Geometry: final body of the model. Coordinates: model frame, mm. Face numbers are marked on the shaded views. A direction names the side the tool comes from. Give positions to 0.01 mm unless a question says otherwise; leave off trailing zeros. Write each loop counter-clockwise with the first axis right and the second up, starting at its lowest first coordinate (ties: lowest second). Pieces come first, ordered by that corner, then holes. Notation, with made-up numbers: M 61,-39.75 L 67,-39.75 A14 cw 67,-12.75 Z; hole C 86.25,89 d11. An arc over 180 degrees is marked long. Use a Markdown table: item, result. Add a question column.
1) Section C-C on x = -102.5. Return the cut outline in (y, z).
2) Line query: line 1 (Z direction, x = 0, y = 80); line 2 (Y direction, x = -79.5, z = -69.5); line 3 (X direction, y = 38.5, z = -42). Output: solid intervals per line, ascending.
3) Section A-A on z = -40.5. Return the cut outline in (x, y), then the cut area to 3 significant figures.
4) Section B-B on y = 17. Return the cut outline in (x, z), then the cut area to 3 significant figures.
5) Section D-D on z = -99.5. Return the cut outline in (x, y).
6) Pin query (flat end, axial travel): pin 1 (2 mm diameter, centred on y = 37.5, z = -42, fed in from -X); pin 2 (7.5 mm diameter, centred on x = -71.63, z = -2.45, fed in from -Y); pin 3 (12 mm diameter, centred on y = 24, z = -75.5, fed in from +X). Return the tip coordinate at first contact, or that it passes through.
7) Set-up query: the marked faces 1 and 2. Return all of +Z, -Z, +X, -X, +Y, -Y with unobstructed straight access to the full face (end or side cutting, diameter ignored); none if empty.
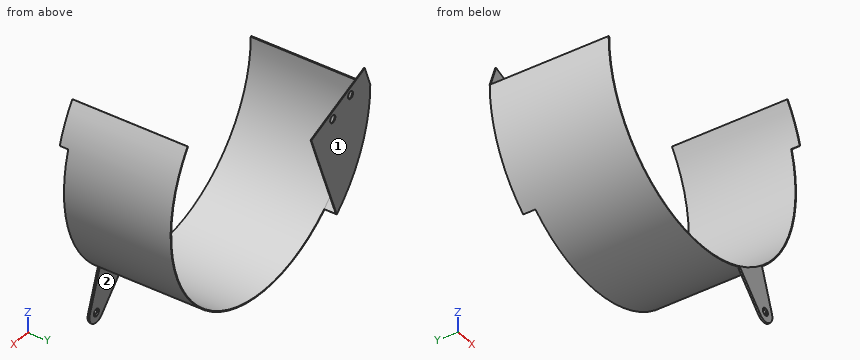
```python
from build123d import *
from build123d.topology import SkipClean

# Parameters (mm, degrees)
BASE_FLANGE1_DEPTH   = 102.87
CUT_EXTRUDE1_START   = -7.62
CUT_EXTRUDE1_DEPTH   = 7.62
BOSS_EXTRUDE5_START  = -95.25
BOSS_EXTRUDE5_DEPTH  = 95.25
BOSS_EXTRUDE6_DEPTH  = 10.16
BOSS_EXTRUDE7_DEPTH  = 0.762
SKETCH12_W           = 72.378245623
SKETCH12_H           = 0.762
BOSS_EXTRUDE8_DEPTH  = 20.33854962
SKETCH13_R           = 3.3
CUT_EXTRUDE2_DEPTH   = 204.597121983
SKETCH15_R           = 3.2639
BOSS_EXTRUDE10_DEPTH = 1.5875


# Read off the part's stored shape, not the designer's step: Cut-Extrude1
# Sheet-metal steps are written as plain solids
with BuildPart() as part:
    # Sketch2 → Base-Flange1 (new body)
    with BuildSketch(Plane(origin=(0, 0, 0), x_dir=(1, 0, 0), z_dir=(0, 1, 0))):
        with BuildLine():
            ThreePointArc((-119.38, 0), (35.898258345, 113.85472958), (97.790371047, -68.473554972))
            Line((97.790371047, -68.473554972), (97.186983651, -68.051058569))
            ThreePointArc((97.186983651, -68.051058569), (35.676758453, 113.152221674), (-118.6434, 0))
            Line((-118.6434, 0), (-119.38, 0))
        make_face()
    extrude(amount=BASE_FLANGE1_DEPTH)

    # Cut-Extrude1 outline → Cut-Extrude1 (cut)
    with BuildSketch(Plane.XZ.offset(CUT_EXTRUDE1_START)):
        with BuildLine():
            ThreePointArc((-119.38, 0), (18.160489843, -117.990597119), (113.85472958, 35.898258345))
            Line((113.85472958, 35.898258345), (113.152221674, 35.676758453))
            ThreePointArc((113.152221674, 35.676758453), (18.048435757, -117.262570031), (-118.6434, 0))
            Line((-118.6434, 0), (-119.38, 0))
        make_face()
    extrude(amount=CUT_EXTRUDE1_DEPTH, mode=Mode.SUBTRACT)

    # Sketch9 → Boss-Extrude5 (add)
    with BuildSketch(Plane(origin=(0, 102.87, 0), x_dir=(1, 0, 0), z_dir=(0, 1, 0)).offset(BOSS_EXTRUDE5_START)):
        with BuildLine():
            Line((-119.379693576, -0.270484204), (-118.6434, 0))
            Line((-118.6434, 0), (-119.38, 0))
            ThreePointArc((-119.38, 0), (-119.379923394, -0.135242189), (-119.379693576, -0.270484204))
        make_face()
    extrude(amount=BOSS_EXTRUDE5_DEPTH)

    # Sketch10 → Boss-Extrude6 (add)
    with SkipClean():  # the faces are left unmerged after this step: merging them gives an invalid solid
        with BuildSketch(Plane(origin=(0, 102.87, 0), x_dir=(1, 0, 0), z_dir=(0, 1, 0))):
            with BuildLine():
                Line((-119.379693576, -0.270484204), (-118.6434, 0))
                ThreePointArc((-118.6434, 0), (-107.527437301, 50.140867475), (-76.262507491, 90.886117283))
                Line((-76.262507491, 90.886117283), (-76.735984844, 91.45038562))
                ThreePointArc((-76.735984844, 91.45038562), (-108.252110006, 50.329564663), (-119.379693576, -0.270484204))
            make_face()
        extrude(amount=BOSS_EXTRUDE6_DEPTH)

    # Sketch11 → Boss-Extrude7 (add)
    with SkipClean():  # the faces are left unmerged after this step: merging them gives an invalid solid
        with BuildSketch(Plane(origin=(0, 113.03, 0), x_dir=(1, 0, 0), z_dir=(0, 1, 0))):
            with BuildLine():
                Line((-119.379693576, -0.270484204), (-51.440692331, 24.687531528))
                Line((-51.440692331, 24.687531528), (-76.735984844, 91.45038562))
                ThreePointArc((-76.735984844, 91.45038562), (-108.252110006, 50.329564663), (-119.379693576, -0.270484204))
            make_face()
        extrude(amount=BOSS_EXTRUDE7_DEPTH)

    # Sketch12 → Boss-Extrude8 (add)
    with SkipClean():  # the faces are left unmerged after this step: merging them gives an invalid solid
        with BuildSketch(Plane(origin=(-14.107419738, 0, -38.402251904), x_dir=(0.9386660406079884, 0, -0.3448275862069655), z_dir=(0.3448275862069655, 0, 0.9386660406079884))):
            with Locations((-75.961811901, 113.411)):
                Rectangle(SKETCH12_W, SKETCH12_H)
        extrude(amount=BOSS_EXTRUDE8_DEPTH)

    # Sketch13 → Cut-Extrude2 (cut, through all)
    with SkipClean():  # the faces are left unmerged after this step: merging them gives an invalid solid
        with BuildSketch(Plane(origin=(0, 113.792, 0), x_dir=(1, 0, 0), z_dir=(0, 1, 0))):
            with Locations(Location((-94.258662261, -5.860928581, 0), (0, 0, 270))):
                Circle(SKETCH13_R)
            with Locations(Location((-71.633967235, 2.450493285, 0), (0, 0, 270))):
                Circle(SKETCH13_R)
        extrude(amount=-CUT_EXTRUDE2_DEPTH, mode=Mode.SUBTRACT)

    # Sketch15 → Boss-Extrude10 (add)
    with SkipClean():  # the faces are left unmerged after this step: merging them gives an invalid solid
        with BuildSketch(Plane.XZ.offset(-7.62)):
            with BuildLine():
                Line((76.054879624, -92.017605302), (88.669451617, -127.404882133))
                ThreePointArc((88.669451617, -127.404882133), (84.957156503, -137.959730204), (73.860989671, -136.524099874))
                Line((73.860989671, -136.524099874), (47.938477772, -109.332002401))
                ThreePointArc((47.938477772, -109.332002401), (62.598204897, -101.651606695), (76.054879624, -92.017605302))
            make_face()
            with Locations(Location((80.295588053, -130.389929705, 0), (0, 0, 270))):
                Circle(SKETCH15_R, mode=Mode.SUBTRACT)
        extrude(amount=-BOSS_EXTRUDE10_DEPTH)


solid = part.part
```
Found:
| question | item | result |
|---|---|---|
| 1 | outline | M 7.62,-61.2 L 113.79,-61.2 L 113.79,15.74 L 113.03,15.74 L 113.03,-59.75 L 7.62,-59.75 Z |
| 2 | line 1 | -119.38 to -118.64 |
| 2 | line 2 | 113.03 to 113.79 |
| 2 | line 3 | -111.75 to -110.96, 110.96 to 111.75 |
| 3 | outline | M -112.3,7.62 L -111.52,7.62 L -111.52,113.03 L -57.43,113.03 L -57.43,113.79 L -112.3,113.79 Z; M 111.52,7.62 L 112.3,7.62 L 112.3,102.87 L 111.52,102.87 Z |
| 3 | area | 199 mm² |
| 4 | outline | M -119.38,0 A119.38 ccw long 97.79,68.47 L 97.19,68.05 A118.64 cw long -118.64,0 L -119.38,0.27 A119.38 ccw Z |
| 4 | area | 329 mm² |
| 5 | outline | M -65.96,7.62 L -64.62,7.62 L -64.62,102.87 L -65.96,102.87 Z; M 64.62,7.62 L 78.72,7.62 L 78.72,9.21 L 65.96,9.21 L 65.96,102.87 L 64.62,102.87 Z |
| 6 | pin 1 | x = -112.12 |
| 6 | pin 2 | y = 113.03 |
| 6 | pin 3 | x = 97.06 |
| 7 | face 1 | +Z, -Z, +X, -X, +Y |
| 7 | face 2 | -Z, +X, +Y |
